Check sheet for the modelled part. Datum: model origin and axes. Units: mm. A direction names the side the tool comes from. Give positions to 0.01 mm unless a question says otherwise; leave off trailing zeros. Write each loop counter-clockwise with the first axis right and the second up, starting at its lowest first coordinate (ties: lowest second). Pieces come first, ordered by that corner, then holes. Notation, with made-up numbers: (-18, 45) -> (26, 45) arc R15 cw to (26, 52) -> close; hole circle Ø10 at (-7.75, -25). An arc over 180 degrees is marked (long way). Answer as a JSON object with one key per item and string values.
from build123d import *

# Parameters (mm, degrees)
F0_R     = 15
F1_DEPTH = 10
F3_R     = 9.15
F4_DEPTH = 10
F5_R     = 5


with BuildPart() as f1:
    # F0 (on Top) → F1 (new body)
    with BuildSketch(Plane.XY):
        Circle(F0_R)
    extrude(amount=F1_DEPTH)

    # F3 (on offset) → F4 (join)
    with BuildSketch(Plane.XY.offset(10)):
        Circle(F3_R)
    extrude(amount=F4_DEPTH)

    # F5
    f5_edges = [f1.edges().sort_by_distance(p)[0] for p in [
        (-15, 0, 0),
    ]]
    fillet(f5_edges, radius=F5_R)


solid = f1.part
1. Access from +Z, -Z, +X, -X, +Y, -Y to the whole of each face (thin tool, end or side, straight path). Record for faces 1 (the face through (0, 0, 20)), 2 (the face through (6.5, 6.9, 10)).
Determined:
{"face 1": "+Z, +X, -X, +Y, -Y", "face 2": "+Z"}
2. Sectioned sample at C-C, the plane z = 6.75. Enter the section's corners in (x, y).
Determined:
{"outline": "circle Ø30 at (0, 0)"}
3. Sectioned sample at A-A, the plane y = 0. Enter the section's corners in (x, z).
Determined:
{"outline": "(-15, 5) arc R5 ccw to (-10, 0) -> (10, 0) arc R5 ccw to (15, 5) -> (15, 10) -> (9.15, 10) -> (9.15, 20) -> (-9.15, 20) -> (-9.15, 10) -> (-15, 10) -> close"}
4. Go/stop test with flat-tipped pins: P1, Ø1, axis at y = -12, z = 2.5, coming from the +X side; P2, Ø5, axis at y = -6.5, z = 5, coming from the +X side; P3, Ø10, axis at x = 2, z = 18, coming from the -Y side. Record where each tip stops, or that it passes through.
Determined:
{"P1": "x = 8.69", "P2": "x = 14.46", "P3": "y = -9.15"}
5. Scan lines: L1, parallel to Y at x = -0.5, z = 5.75; L2, parallel to Z at x = -8, y = 4.75; L3, parallel to Y at x = 2, z = 17.75. Record each from-to range of solid material in increasing order. Write a range as [from, to].
Determined:
{"L1": "[-14.99, 14.99]", "L2": "[0, 10]", "L3": "[-8.93, 8.93]"}
6. Sectioned sample at D-D, the plane z = 15. Enter the section's corners in (x, y), plus the area to 3 significant figures.
Determined:
{"outline": "circle Ø18.3 at (0, 0)", "area": "263 mm^2"}
